The model under review builds one solid part; all positions refer to its coordinate system, in mm. A direction names the side the tool comes from. Give positions to 0.01 mm unless a question says otherwise; leave off trailing zeros. Loops run counter-clockwise (first coordinate to the right, second up) from the corner with the lowest first, then second, coordinate; pieces in that order, holes last. Notation, with made-up numbers: (-35.75, 31) -> (8.25, 31) arc R16 ccw to (8.25, 54) -> close; hole circle Ø6 at (66, 73). An arc over 180 degrees is marked (long way). Write each question's results on one line, items separated by ' | '. Start each with the question number.
Q1. We need section D-D (y = 50.8). Write out the cut boundary in (x, z), plus the area to 3 significant figures.
Q2. Mouldability with a two-part tool opening along X and no side actions: class faces 3 (the face through (-11.3, -63.5, 7.1)), 4 (the face through (-11.112, -1, 13)), 5 (the face through (-8.4, -51.71, 0.78)) as released by +X, released by -X, zero draft, split by the parting line, or undercut.
Q3. We need section A-A (y = 31.75). Write out the cut boundary in (x, z).
Q4. Machinability: for faces 1 (the face through (1, -1, 1.588)), 2 (the face through (-12.7, -1, 13)), which of the approach directions +Z, -Z, +X, -X, +Y, -Y give a long, thin tool a straight path to every point of the face, cutting with its end or side? Answer none if there is none.
Q5. We need section B-B (x = 0). Write out the cut boundary in (y, z).
Q6. Wall thickness on L1, parallel to X at y = -50.8, z = 0.8; L2, parallel to Z at x = 7, y = 27; L3, parallel to X at y = 42.5, z = 12.75: over which ranges is each line inside the solid? List them lowest first. Write a range as [from, to].
Q7. Insertion check: pin 1 Ø3.5 at (x, y) = (8.98, -50.8) entering from +Z; pin 2 Ø4 at (x, y) = (8, 5.5) entering from -Z; pin 3 Ø12 at (y, z) = (1, 10.5) entering from +X. Each pin has a flat end and moves straight along its axis. Give the tip position at first contact, or say it passes through.
Q8. We need section C-C (z = 12.7). Write out the cut boundary in (x, y), plus the area to 3 significant figures.
from build123d import *

# Parameters (mm, degrees)
F2_DEPTH = 63.5
F0_R     = 7.3279
F0_R_2   = 1.0795
F3_DEPTH = 25.401
F4_R     = 2.0955
F5_DEPTH = 25.401


with BuildPart() as f2:
    # F1 (on Front) → F2 (new body, symmetric)
    with BuildSketch(Plane.XZ):
        Polygon((12.7, 0), (12.7, 1.5875), (-11.1125, 1.5875), (-11.1125, 25.4), (-12.7, 25.4), (-12.7, 0), align=None)
    extrude(amount=F2_DEPTH, both=True)


with BuildPart() as f3:
    # F0 (on Top) → F3 (new body, through all)
    with BuildSketch(Plane.XY):
        with Locations((0, 50.8)):
            Circle(F0_R)
        with Locations((0, 59.780256)):
            Circle(F0_R_2)
        with Locations((8.980256, 50.8)):
            Circle(F0_R_2)
        with Locations((0, 41.819744)):
            Circle(F0_R_2)
        with Locations((-8.980256, 50.8)):
            Circle(F0_R_2)
    extrude(amount=F3_DEPTH)


with BuildPart() as f5:
    # F4 (on face) → F5 (new body, through all)
    with BuildSketch(Plane(origin=(-12.7, 0, 0), x_dir=(0, -1, 0), z_dir=(-1, 0, 0))):
        with Locations((-31.75, 12.7)):
            Circle(F4_R)
    extrude(amount=-F5_DEPTH)


with BuildPart() as f6_1:
    # F6: instance of F3
    add(f3.part.mirror(Plane.XZ))


with BuildPart() as f6_2:
    # F6: instance of F5
    add(f5.part.mirror(Plane.XZ))


with BuildPart() as f2_1:
    add(f2.part)

    # F7: cut F5, F6_2, F3, F6_1
    add(f5.part, mode=Mode.SUBTRACT)
    add(f6_2.part, mode=Mode.SUBTRACT)
    add(f3.part, mode=Mode.SUBTRACT)
    add(f6_1.part, mode=Mode.SUBTRACT)


solid = f2_1.part
Output:
1) outline: (-12.7, 0) -> (-10.06, 0) -> (-10.06, 1.59) -> (-11.11, 1.59) -> (-11.11, 25.4) -> (-12.7, 25.4) -> close; (-7.9, 0) -> (-7.33, 0) -> (-7.33, 1.59) -> (-7.9, 1.59) -> close; (7.33, 0) -> (7.9, 0) -> (7.9, 1.59) -> (7.33, 1.59) -> close; (10.06, 0) -> (12.7, 0) -> (12.7, 1.59) -> (10.06, 1.59) -> close | area: 48.0 mm2
2) face 3: zero draft | face 4: released by +X | face 5: undercut
3) outline: (-12.7, 0) -> (12.7, 0) -> (12.7, 1.59) -> (-11.11, 1.59) -> (-11.11, 10.6) -> (-12.7, 10.6) -> close; (-12.7, 14.8) -> (-11.11, 14.8) -> (-11.11, 25.4) -> (-12.7, 25.4) -> close
4) face 1: +Z, +X, +Y, -Y | face 2: +Z, -Z, -X, +Y, -Y
5) outline: (-63.5, 0) -> (-60.86, 0) -> (-60.86, 1.59) -> (-63.5, 1.59) -> close; (-58.7, 0) -> (-58.13, 0) -> (-58.13, 1.59) -> (-58.7, 1.59) -> close; (-43.47, 0) -> (-42.9, 0) -> (-42.9, 1.59) -> (-43.47, 1.59) -> close; (-40.74, 0) -> (40.74, 0) -> (40.74, 1.59) -> (-40.74, 1.59) -> close; (42.9, 0) -> (43.47, 0) -> (43.47, 1.59) -> (42.9, 1.59) -> close; (58.13, 0) -> (58.7, 0) -> (58.7, 1.59) -> (58.13, 1.59) -> close; (60.86, 0) -> (63.5, 0) -> (63.5, 1.59) -> (60.86, 1.59) -> close
6) L1: [-12.7, -10.06], [-7.9, -7.33], [7.33, 7.9], [10.06, 12.7] | L2: [0, 1.59] | L3: [-12.7, -11.11]
7) pin 1: z = 1.59 | pin 2: z = 0 | pin 3: x = -11.11
8) outline: (-12.7, -63.5) -> (-11.11, -63.5) -> (-11.11, -33.85) -> (-12.7, -33.85) -> close; (-12.7, -29.65) -> (-11.11, -29.65) -> (-11.11, 29.65) -> (-12.7, 29.65) -> close; (-12.7, 33.85) -> (-11.11, 33.85) -> (-11.11, 63.5) -> (-12.7, 63.5) -> close | area: 188 mm2
